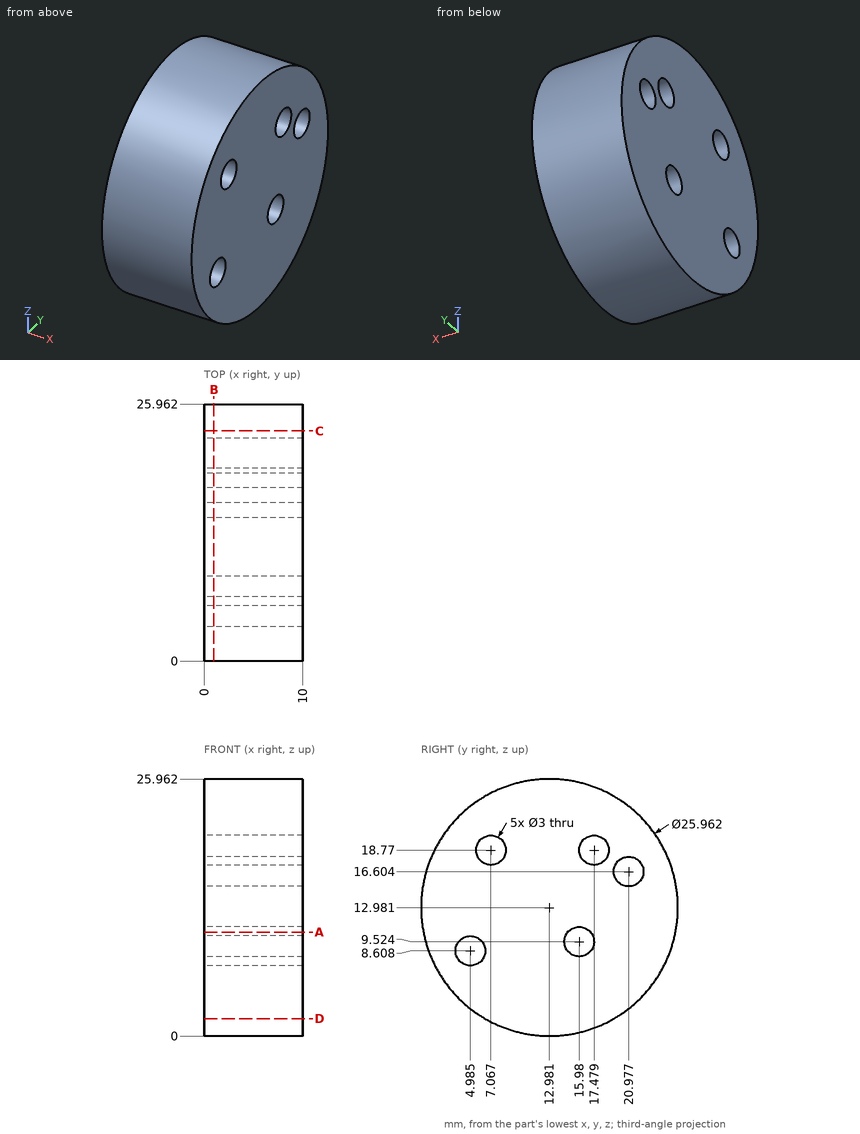
Answer from the drawing. Dimensions are ordinates in mm from the lowest x, y and z of the part. Round coordinates to 2 decimals unless told otherwise and drop trailing zeros. Order: outer loops, then holes, each group sorted by start corner. A loop starts at its lowest first (then second) coordinate and runs counter-clockwise, first axis right, second up.
1) The part is cut by section B-B on x = 1. Write down the section's boundary in (y, z) (1 decimal), plus the area to 3 significant figures.
2) The part is cut by section C-C on y = 23.25. Write down the section's boundary in (x, z).
3) Flat-ended cylindrical pins translate along their axes: pin 1 (3.5 mm diameter, centred on y = 20.98, z = 16.6, fed in from -X); pin 2 (2 mm diameter, centred on x = 2.5, y = 8.5, fed in from -Z) (1 decimal); pin 3 (5 mm diameter, centred on x = 4, z = 21.5, fed in from +Y). Find the tip coordinate at first contact, or state that the pin passes through.
4) Straight lines are drawn through the part: L1, parallel to Y at x = 4.5, z = 17.75 (1 decimal); L2, parallel to Y at x = 0.5, z = 18.25 (1 decimal); L3, parallel to Z at x = 0.5, y = 18.5. For each, find the intervals that lie inside material, in ascending order.
5) The part is cut by section A-A on z = 10.5. Write down the section's boundary in (x, y).
6) The part is cut by section D-D on z = 1.75. Write down the section's boundary in (x, y).
Resolved:
1. outline: circle Ø26 at (13, 13); hole circle Ø3 at (5, 8.6); hole circle Ø3 at (7.1, 18.8); hole circle Ø3 at (16, 9.5); hole circle Ø3 at (17.5, 18.8); hole circle Ø3 at (21, 16.6)
1. area: 494 mm2
2. outline: (0, 5.04) - (10, 5.04) - (10, 20.92) - (0, 20.92) - close
3. pin 1: stops at x = 0
3. pin 2: stops at z = 0.5
3. pin 3: stops at y = 24.48
4. L1: y = 0.9 to 6, 8.2 to 16.4, 18.6 to 20, 21.9 to 25.1
4. L2: y = 1.1 to 5.7, 8.5 to 16.1, 18.9 to 24.8
4. L3: z = 1.23 to 17.67, 19.87 to 24.73
5. outline: (0, 0.24) - (10, 0.24) - (10, 14.84) - (0, 14.84) - close; (0, 17.12) - (10, 17.12) - (10, 25.72) - (0, 25.72) - close
6. outline: (0, 6.47) - (10, 6.47) - (10, 19.49) - (0, 19.49) - close
